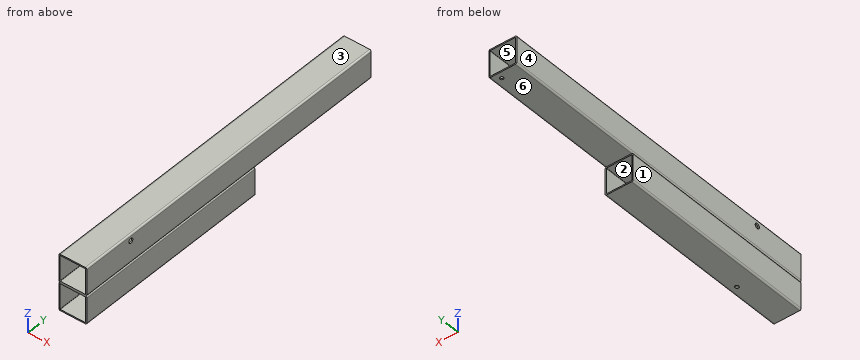
from build123d import *

# Parameters (mm, degrees)
F1_DEPTH = 1100
F2_R     = 8
F3_DEPTH = 90.001
F4_W     = 450
F4_H     = 80
F4_H_2   = 5
F5_DEPTH = 90.001
F6_R     = 6
F7_DEPTH = 4
F8_R     = 6
F9_DEPTH = 4


with BuildPart() as f1:
    # F0 (on Front) → F1 (new body)
    with BuildSketch(Plane.XZ):
        with BuildLine():
            ThreePointArc((45, 40), (43.5355339059, 43.5355339059), (40, 45))
            Line((40, 45), (-40, 45))
            ThreePointArc((-40, 45), (-43.5355339059, 43.5355339059), (-45, 40))
            Line((-45, 40), (-45, -40))
            ThreePointArc((-45, -40), (-43.5355339059, -43.5355339059), (-40, -45))
            Line((-40, -45), (40, -45))
            ThreePointArc((40, -45), (43.5355339059, -43.5355339059), (45, -40))
            Line((45, -40), (45, 40))
        make_face()
        with BuildLine():
            ThreePointArc((-41, 40), (-40.7071067812, 40.7071067812), (-40, 41))
            Line((-40, 41), (40, 41))
            ThreePointArc((40, 41), (40.7071067812, 40.7071067812), (41, 40))
            Line((41, 40), (41, -40))
            ThreePointArc((41, -40), (40.7071067812, -40.7071067812), (40, -41))
            Line((40, -41), (-40, -41))
            ThreePointArc((-40, -41), (-40.7071067812, -40.7071067812), (-41, -40))
            Line((-41, -40), (-41, 40))
        make_face(mode=Mode.SUBTRACT)
        with BuildLine():
            ThreePointArc((45, -50), (43.5355339059, -46.4644660941), (40, -45))
            Line((40, -45), (-40, -45))
            ThreePointArc((-40, -45), (-43.5355339059, -46.4644660941), (-45, -50))
            Line((-45, -50), (-45, -130))
            ThreePointArc((-45, -130), (-43.5355339059, -133.5355339059), (-40, -135))
            Line((-40, -135), (40, -135))
            ThreePointArc((40, -135), (43.5355339059, -133.5355339059), (45, -130))
            Line((45, -130), (45, -50))
        make_face()
        with BuildLine():
            ThreePointArc((-41, -50), (-40.7071067812, -49.2928932188), (-40, -49))
            Line((-40, -49), (40, -49))
            ThreePointArc((40, -49), (40.7071067812, -49.2928932188), (41, -50))
            Line((41, -50), (41, -130))
            ThreePointArc((41, -130), (40.7071067812, -130.7071067812), (40, -131))
            Line((40, -131), (-40, -131))
            ThreePointArc((-40, -131), (-40.7071067812, -130.7071067812), (-41, -130))
            Line((-41, -130), (-41, -50))
        make_face(mode=Mode.SUBTRACT)
    extrude(amount=-F1_DEPTH)

    # F2 (on face) → F3 (cut, through all)
    with BuildSketch(Plane.YZ.offset(45)):
        with Locations((170, 25)):
            Circle(F2_R)
    extrude(amount=-F3_DEPTH, mode=Mode.SUBTRACT)

    # F4 (on face) → F5 (cut, through all)
    with BuildSketch(Plane.YZ.offset(45)):
        with Locations((875, -90)):
            Rectangle(F4_W, F4_H)
        with Locations((875, -47.5)):
            Rectangle(F4_W, F4_H_2)
        with Locations((875, -132.5)):
            Rectangle(F4_W, F4_H_2)
    extrude(amount=-F5_DEPTH, mode=Mode.SUBTRACT)

    # F6 (on face) → F7 (cut, through all)
    with BuildSketch(Plane(origin=(0, 0, -135), x_dir=(1, 0, 0), z_dir=(0, 0, -1))):
        with Locations((20, -170)):
            Circle(F6_R)
    extrude(amount=-F7_DEPTH, mode=Mode.SUBTRACT)

    # F8 (on face) → F9 (cut, through all)
    with BuildSketch(Plane(origin=(0, 0, -45), x_dir=(1, 0, 0), z_dir=(0, 0, -1))):
        with Locations((20, -1080)):
            Circle(F8_R)
    extrude(amount=-F9_DEPTH, mode=Mode.SUBTRACT)


solid = f1.part
Build history of the part. All positions in model axes, mm. Face numbers are marked on the shaded views. A direction names the side the tool comes from. Round coordinates to 2 decimals unless told otherwise and drop trailing zeros. Write each loop counter-clockwise with the first axis right and the second up, starting at its lowest first coordinate (ties: lowest second). Pieces come first, ordered by that corner, then holes. Notation, with made-up numbers: (22, 7.5) - (42, 7.5) arc R26 cw to (42, 36.5) - close; hole circle Ø7 at (1.5, 8). An arc over 180 degrees is marked (long way). Use CSV: the item, a comma, the result in double quotes.
(1) Wall check: line 1 (Z direction, x = 38, y = 474.5); line 2 (Y direction, x = 20, z = -132.35); line 3 (X direction, y = 811.5, z = 35). Give the ranges that are in metal, low to high.
Response:
line 1,"-135 to -131, -49 to -41, 41 to 45"
line 2,"0 to 164, 176 to 650"
line 3,"-45 to -41, 41 to 45"
(2) 3-axis set-ups, long thin cutter, end or side, ignore diameter. For the marked faces 4, 5 and 6: which of +Z, -Z, +X, -X, +Y, -Y reach the whole face in a straight line?
Response:
face 4,"+Z, -Z, -X, +Y, -Y"
face 5,"+Y, -Y"
face 6,"-Z, +X, -X, +Y"
(3) Mould opens along Z. For the marked faces 1, 2 and 3 say: pulls with the +Z half, pulls with the -Z half, needs draft (parallel to the pull), parting line crosses it, or undercut.
Response:
face 1,"needs draft"
face 2,"undercut"
face 3,"pulls with the +Z half"
(4) Band-saw the part on C-C (y = 313). Give the number of separate pieces and of enclosed holes in the cut face, plus the area to 3 significant figures.
Response:
separate pieces,"1"
enclosed holes,"2"
area,"2,710 mm²"
(5) Pin check, flat tips, straight feed: P1, Ø1, axis at x = 30, y = 759.5, coming from the -Z side; P2, Ø11, axis at x = 20, y = 1080, coming from the -Z side. Stop position of each tip, or through.
Response:
P1,"z = -45"
P2,"z = 41"
(6) Band-saw the part on A-A (x = 2). Write the cut outline in (y, z), plus the area to 3 significant figures.
Response:
outline,"(0, -135) - (650, -135) - (650, -131) - (0, -131) - close; (0, -49) - (650, -49) - (650, -45) - (1100, -45) - (1100, -41) - (0, -41) - close; (0, 41) - (1100, 41) - (1100, 45) - (0, 45) - close"
area,"14,000 mm²"
(7) Band-saw the part on B-B (z = -10). Write the cut outline in (x, y).
Response:
outline,"(-45, 0) - (-41, 0) - (-41, 1100) - (-45, 1100) - close; (41, 0) - (45, 0) - (45, 1100) - (41, 1100) - close"
(8) Band-saw the part on D-D (y = 1012). Write the cut outline in (x, z).
Response:
outline,"(-45, -40) arc R5 ccw to (-40, -45) - (40, -45) arc R5 ccw to (45, -40) - (45, 40) arc R5 ccw to (40, 45) - (-40, 45) arc R5 ccw to (-45, 40) - close; hole (-41, -40) arc R1 ccw to (-40, -41) - (40, -41) arc R1 ccw to (41, -40) - (41, 40) arc R1 ccw to (40, 41) - (-40, 41) arc R1 ccw to (-41, 40) - close"
